Read the model definition and answer for the solid it produces. Units are mm, in the model's axes. A direction names the side the tool comes from. Coordinates: 2 decimals unless noted, no trailing zeros. Order: outer loops, then holes, each group sorted by start corner. A loop starts at its lowest first (then second) coordinate and runs counter-clockwise, first axis right, second up. Notation, with made-up numbers: M 71,60 L 75,60 A21 ccw 75,72 Z; hole C -25.5,29 d8. An arc over 180 degrees is marked long. Use a Markdown table: item, result. Add a question column.
1) Each of these flat-tipped pins is pushed along its axis until it touches: pin 1 Ø2 at (y, z) = (-5.5, -84) entering from +X; pin 2 Ø4 at (x, y) = (426, -11) entering from -Z; pin 3 Ø1 at (y, z) = (-2, -69.5) entering from -X. Where does it stop, or does it pass through?
2) Find the intervals of material crossed by probe 1 along X at (y, z) = (-1, -14); probe 2 along X at (y, z) = (13, -69.5); probe 3 along Y at (x, z) = (1145, -97), in increasing order. Write a range as [from, to].
3) For faces 1 (the face through (23.846, -7.509, -25.35)), 2 (the face through (0, 0, 0)), determine the directions among +Z, -Z, +X, -X, +Y, -Y from which every point of the face is accessible in a straight line to the end or side of a thin tool.
4) Find section A-A on z = -25.5. Write down the section's boundary in (x, y).
from build123d import *

# Parameters (mm, degrees)
SKETCH2_R = 25


with BuildPart() as part:
    # Sweep1: sweep along a path in Sketch1
    with BuildLine(Plane(origin=(0, 0, 0), x_dir=(1, 0, 0), z_dir=(0, 1, 0))) as sweep1_path:
        Line((0, 0), (0, 50))
        ThreePointArc((0, 50), (14.644660941, 85.355339059), (50, 100))
        Line((50, 100), (1228.6, 100))
        ThreePointArc((1228.6, 100), (1263.955339059, 85.355339059), (1278.6, 50))
        Line((1278.6, 50), (1278.6, 0))
    # Sketch2 → Sweep1 (sweep)
    with BuildSketch(Plane.XY):
        Circle(SKETCH2_R)
    sweep(path=sweep1_path.line)


solid = part.part
Check result:
| question | item | result |
|---|---|---|
| 1 | pin 1 | stops at x = 1295.32 |
| 1 | pin 2 | stops at z = -123.32 |
| 1 | pin 3 | stops at x = -22.48 |
| 2 | probe 1 | x = [-24.98, 24.98], [1253.62, 1303.58] |
| 2 | probe 2 | x = [-18.64, 29.02], [1249.58, 1297.24] |
| 2 | probe 3 | y = [-24.82, 24.82] |
| 3 | face 1 | +Z |
| 3 | face 2 | +Z, +X, -X, +Y, -Y |
| 4 | outline | C 0,0 d50; C 1278.6,0 d50 |
